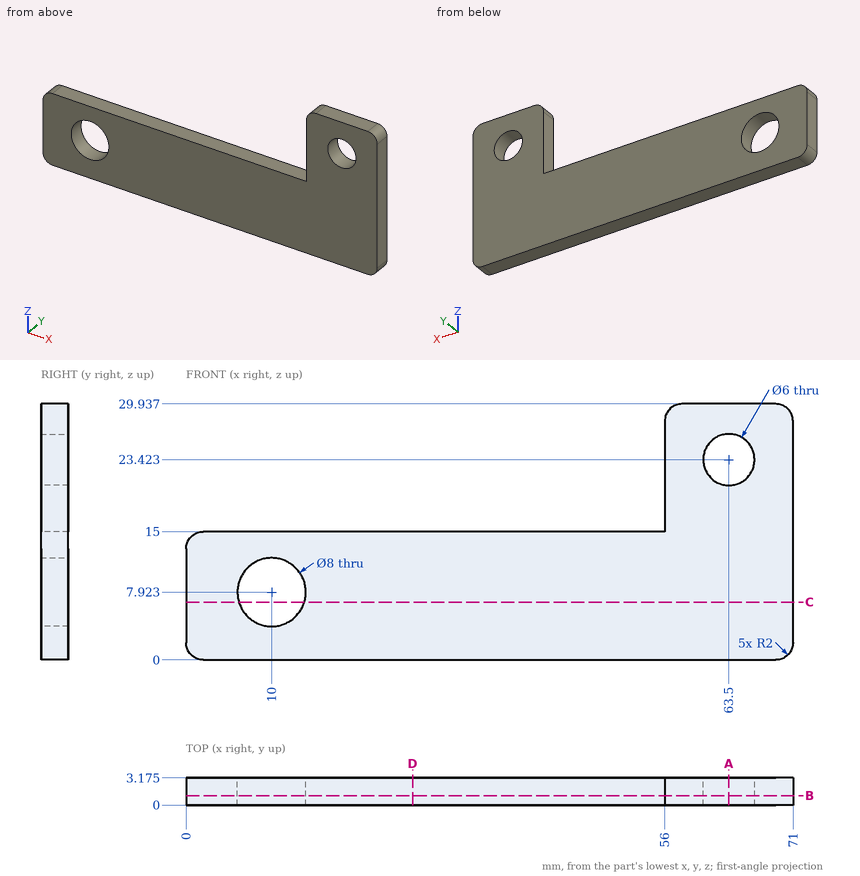
Job drawing, mm, ordinate dimensions from the low corner. One solid piece. Give positions to 0.01 mm unless a question says otherwise; leave off trailing zeros. Order: outer loops, then holes, each group sorted by start corner. A loop starts at its lowest first (then second) coordinate and runs counter-clockwise, first axis right, second up. Notation, with made-up numbers: M -4.5,40 L 49.5,40 A23 ccw 49.5,53 Z; hole C -36.75,89 d1. An arc over 180 degrees is marked long. Put each result on its own line as item: value. Start each with the question number.
(1) Band-saw the part on A-A on x = 63.5. Give the cut face in (y, z) (1 decimal).
(2) Pin check, flat tip, straight feed: pin 1 Ø4 at (x, z) = (40, 8.5) entering from -Y. Stop position of the tip, or through.
(3) Band-saw the part on B-B on y = 1.1. Give the cut face in (x, z), then the cut area to 3 significant figures.
(4) Drill centre lines: L1, parallel to X at y = 2.75, z = 8; L2, parallel to Z at x = 44, y = 1.4; L3, parallel to X at y = 0.3, z = 27.25. Where is each one in solid material? Low to high. Write a range as [from, to].
(5) Band-saw the part on D-D on x = 26.5. Give the cut face in (y, z) (1 decimal).
(6) Band-saw the part on C-C on z = 6.75. Give the cut face in (x, y) (1 decimal).
Results below:
1. outline: M 0,0 L 3.2,0 L 3.2,20.4 L 0,20.4 Z; M 0,26.4 L 3.2,26.4 L 3.2,29.9 L 0,29.9 Z
2. pin 1: stops at y = 0
3. outline: M 0,2 A2 ccw 2,0 L 69,0 A2 ccw 71,2 L 71,27.94 A2 ccw 69,29.94 L 58,29.94 A2 ccw 56,27.94 L 56,15 L 2,15 A2 ccw 0,13 Z; hole C 10,7.92 d8; hole C 63.5,23.42 d6
3. area: 1,210 mm2
4. L1: x = [0, 6], [14, 71]
4. L2: z = [0, 15]
4. L3: x = [56, 71]
5. outline: M 0,0 L 3.2,0 L 3.2,15 L 0,15 Z
6. outline: M 0,0 L 6.2,0 L 6.2,3.2 L 0,3.2 Z; M 13.8,0 L 71,0 L 71,3.2 L 13.8,3.2 Z
